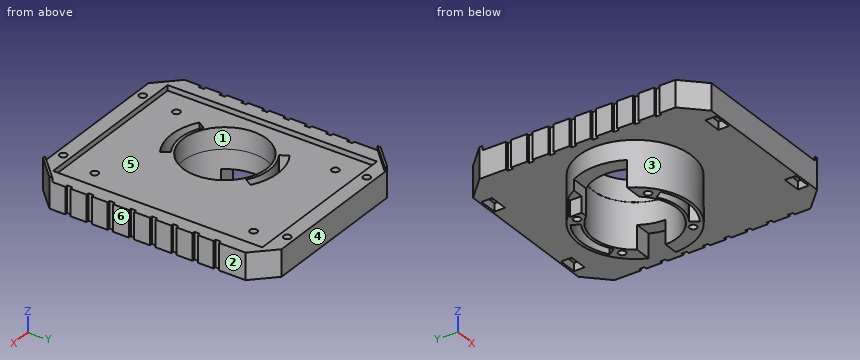
```python
from build123d import *

# Parameters (mm, degrees)
SKETCH1_W           = 92.71
SKETCH1_H           = 114.3
BOSS_EXTRUDE1_DEPTH = 12.7
SKETCH2_W           = 78.71000006
SKETCH2_H           = 100.30000006
CUT_EXTRUDE1_DEPTH  = 2.54
SKETCH3_R           = 19.939
CUT_EXTRUDE2_DEPTH  = 75.284144506
SKETCH4_R           = 26.9875
SKETCH4_R_2         = 19.98750003
BOSS_EXTRUDE2_DEPTH = 21.844
SKETCH6_R           = 1.750000056
CUT_EXTRUDE3_DEPTH  = 19.05
SKETCH12_W          = 12.7
SKETCH12_H          = 25.4
CUT_EXTRUDE6_DEPTH  = 77.759812799
SKETCH13_W          = 11.43
SKETCH13_H          = 11.43
CUT_EXTRUDE7_DEPTH  = 77.759812799
SKETCH14_R          = 1.750000056
CUT_EXTRUDE8_DEPTH  = 82.290814124
SKETCH16_W          = 8.89
SKETCH16_H          = 5.08
CUT_EXTRUDE9_DEPTH  = 3.81
SKETCH18_R          = 1.75
CUT_EXTRUDE11_DEPTH = 5.08
SKETCH19_W          = 2.54
SKETCH19_H          = 2.54
CUT_EXTRUDE12_DEPTH = 82.290814124
CHAMFER2_SIZE       = 10.16
CUT_EXTRUDE13_DEPTH = 82.290814124
BOSS_EXTRUDE3_DEPTH = 2
CUT_EXTRUDE14_START = -7.62
CUT_EXTRUDE14_DEPTH = 7.62


with BuildPart() as part:
    # Sketch1 → Boss-Extrude1 (new body)
    with BuildSketch(Plane.XY):
        Rectangle(SKETCH1_W, SKETCH1_H)
    extrude(amount=BOSS_EXTRUDE1_DEPTH)

    # Sketch2 → Cut-Extrude1 (cut)
    with BuildSketch(Plane.XY.offset(12.7)):
        Rectangle(SKETCH2_W, SKETCH2_H)
    extrude(amount=-CUT_EXTRUDE1_DEPTH, mode=Mode.SUBTRACT)

    # Sketch3 → Cut-Extrude2 (cut, through all)
    with BuildSketch(Plane.XY.offset(10.16)):
        with Locations((-13.335, -4.572)):
            Circle(SKETCH3_R)
    extrude(amount=-CUT_EXTRUDE2_DEPTH, mode=Mode.SUBTRACT)

    # Sketch4 → Boss-Extrude2 (add)
    with BuildSketch(Plane(origin=(0, 0, 0), x_dir=(-1, 0, 0), z_dir=(0, 0, -1))):
        with Locations((13.335, -4.572)):
            Circle(SKETCH4_R)
        with Locations((13.335, -4.572)):
            Circle(SKETCH4_R_2, mode=Mode.SUBTRACT)
    extrude(amount=BOSS_EXTRUDE2_DEPTH)

    # Sketch6 → Cut-Extrude3 (cut)
    with BuildSketch(Plane(origin=(0, 0, -21.844), x_dir=(-1, 0, 0), z_dir=(0, 0, -1))):
        with Locations((-2.11782644, 12.446)):
            Circle(SKETCH6_R)
        with Locations((28.78782644, -21.59)):
            Circle(SKETCH6_R)
        with Locations((28.78782644, 12.446)):
            Circle(SKETCH6_R)
        with Locations((-2.11782644, -21.59)):
            Circle(SKETCH6_R)
    extrude(amount=-CUT_EXTRUDE3_DEPTH, mode=Mode.SUBTRACT)

    # Sketch12 → Cut-Extrude6 (cut, through all)
    with BuildSketch(Plane(origin=(0, 0, 0), x_dir=(0, 0, -1), z_dir=(1, 0, 0))):
        with Locations((15.494, -4.572)):
            Rectangle(SKETCH12_W, SKETCH12_H)
    extrude(amount=-CUT_EXTRUDE6_DEPTH, mode=Mode.SUBTRACT)

    # Sketch13 → Cut-Extrude7 (cut, through all)
    with BuildSketch(Plane(origin=(0, 0, 0), x_dir=(0, 0, -1), z_dir=(1, 0, 0))):
        with Locations((16.129, 0.508)):
            Rectangle(SKETCH13_W, SKETCH13_H)
    extrude(amount=CUT_EXTRUDE7_DEPTH, mode=Mode.SUBTRACT)

    # Sketch14 → Cut-Extrude8 (cut, through all)
    with BuildSketch(Plane.XY.offset(12.7)):
        with Locations((-27.305, 53.65)):
            Circle(SKETCH14_R)
        with Locations((27.305, 53.65)):
            Circle(SKETCH14_R)
        with Locations((-27.305, -53.65)):
            Circle(SKETCH14_R)
        with Locations((27.305, -53.65)):
            Circle(SKETCH14_R)
    extrude(amount=-CUT_EXTRUDE8_DEPTH, mode=Mode.SUBTRACT)

    # Sketch16 → Cut-Extrude9 (cut)
    with BuildSketch(Plane(origin=(0, 0, 0), x_dir=(-1, 0, 0), z_dir=(0, 0, -1))):
        with Locations((-27.305, 53.65)):
            Rectangle(SKETCH16_W, SKETCH16_H)
        with Locations((27.305, 53.65)):
            Rectangle(SKETCH16_W, SKETCH16_H)
        with Locations((27.305, -53.65)):
            Rectangle(SKETCH16_W, SKETCH16_H)
        with Locations((-27.305, -53.65)):
            Rectangle(SKETCH16_W, SKETCH16_H)
    extrude(amount=-CUT_EXTRUDE9_DEPTH, mode=Mode.SUBTRACT)

    # Sketch18 → Cut-Extrude11 (cut)
    with BuildSketch(Plane.XY.offset(10.16)):
        with Locations((-28.17900003, 38.02150003)):
            Circle(SKETCH18_R)
        with Locations((27.92500003, 38.02150003)):
            Circle(SKETCH18_R)
        with Locations((-28.17900003, -38.14850003)):
            Circle(SKETCH18_R)
        with Locations((27.92500003, -38.14850003)):
            Circle(SKETCH18_R)
    extrude(amount=-CUT_EXTRUDE11_DEPTH, mode=Mode.SUBTRACT)

    # Sketch19 → Cut-Extrude12 (cut, through all)
    with BuildSketch(Plane.XY.offset(12.7)):
        with Locations((-46.355, -38.1)):
            Rectangle(SKETCH19_W, SKETCH19_H)
        with Locations((46.355, -38.1)):
            Rectangle(SKETCH19_W, SKETCH19_H)
        with Locations((-46.355, -27.94)):
            Rectangle(SKETCH19_W, SKETCH19_H)
        with Locations((46.355, -27.94)):
            Rectangle(SKETCH19_W, SKETCH19_H)
        with Locations((-46.355, -17.78)):
            Rectangle(SKETCH19_W, SKETCH19_H)
        with Locations((46.355, -17.78)):
            Rectangle(SKETCH19_W, SKETCH19_H)
        with Locations((-46.355, -7.62)):
            Rectangle(SKETCH19_W, SKETCH19_H)
        with Locations((46.355, -7.62)):
            Rectangle(SKETCH19_W, SKETCH19_H)
        with Locations((-46.355, 2.54)):
            Rectangle(SKETCH19_W, SKETCH19_H)
        with Locations((46.355, 2.54)):
            Rectangle(SKETCH19_W, SKETCH19_H)
        with Locations((-46.355, 12.7)):
            Rectangle(SKETCH19_W, SKETCH19_H)
        with Locations((46.355, 12.7)):
            Rectangle(SKETCH19_W, SKETCH19_H)
        with Locations((-46.355, 22.86)):
            Rectangle(SKETCH19_W, SKETCH19_H)
        with Locations((46.355, 22.86)):
            Rectangle(SKETCH19_W, SKETCH19_H)
        with Locations((-46.355, 33.02)):
            Rectangle(SKETCH19_W, SKETCH19_H)
        with Locations((46.355, 33.02)):
            Rectangle(SKETCH19_W, SKETCH19_H)
    extrude(amount=-CUT_EXTRUDE12_DEPTH, mode=Mode.SUBTRACT)

    # Chamfer2
    chamfer2_edges = [part.edges().sort_by_distance(p)[0] for p in [
        (46.355, -57.15, 6.35),
        (-46.355, -57.15, 6.35),
        (-46.355, 57.15, 6.35),
        (46.355, 57.15, 6.35),
    ]]
    chamfer(chamfer2_edges, length=CHAMFER2_SIZE)

    # Sketch20 → Cut-Extrude13 (cut, through all)
    with BuildSketch(Plane(origin=(0, 0, -21.844), x_dir=(-1, 0, 0), z_dir=(0, 0, -1))):
        with BuildLine():
            Line((-0.161794567, 17.099636308), (2.084843313, 13.492237618))
            ThreePointArc((2.084843313, 13.492237618), (13.335, 16.709041004), (24.585156687, 13.492237618))
            Line((24.585156687, 13.492237618), (26.831794567, 17.099636308))
            ThreePointArc((26.831794567, 17.099636308), (13.335, 20.958830066), (-0.161794567, 17.099636308))
        make_face()
        with BuildLine():
            Line((2.084843313, -22.636237618), (-0.161794567, -26.243636308))
            ThreePointArc((-0.161794567, -26.243636308), (13.335, -30.102830066), (26.831794567, -26.243636308))
            Line((26.831794567, -26.243636308), (24.585156687, -22.636237618))
            ThreePointArc((24.585156687, -22.636237618), (13.335, -25.853041004), (2.084843313, -22.636237618))
        make_face()
    extrude(amount=-CUT_EXTRUDE13_DEPTH, mode=Mode.SUBTRACT)

    # Sketch21 → Boss-Extrude3 (add)
    with BuildSketch(Plane.XY.offset(12.7)):
        Polygon((-40.567893219, 51.362893219), (-46.355, 45.575786438), (-46.355, 46.99), (-36.195, 57.15), (-34.780786438, 57.15), align=None)
        Polygon((40.567893219, -51.362893219), (34.780786438, -57.15), (36.195, -57.15), (46.355, -46.99), (46.355, -45.575786438), align=None)
    extrude(amount=BOSS_EXTRUDE3_DEPTH)

    # Sketch22 → Cut-Extrude14 (cut)
    with BuildSketch(Plane(origin=(0, 0, -21.844), x_dir=(-1, 0, 0), z_dir=(0, 0, -1)).offset(CUT_EXTRUDE14_START)):
        with BuildLine():
            Line((31.787826536, 8.128), (31.787826536, 13.716))
            Line((31.787826536, 13.716), (33.181264441, 13.716))
            ThreePointArc((33.181264441, 13.716), (35.342461556, 11.04839667), (37.1475, 8.128))
            Line((37.1475, 8.128), (31.787826536, 8.128))
        make_face()
    extrude(amount=CUT_EXTRUDE14_DEPTH, mode=Mode.SUBTRACT)


solid = part.part
```
For this review, take the finished solid that the model builds, in its own axes (mm). Face numbers are marked on the shaded views. A direction names the side the tool comes from. Round coordinates to 2 decimals unless told otherwise and drop trailing zeros. Write each loop counter-clockwise with the first axis right and the second up, starting at its lowest first coordinate (ties: lowest second). Pieces come first, ordered by that corner, then holes. Notation, with made-up numbers: (13.5, 10.5) -> (68.5, 10.5) arc R15 cw to (68.5, 39.5) -> close; hole circle Ø7 at (-11.75, -29). An arc over 180 degrees is marked (long way). Use one line per item in the form item = value.
1) Take a section at A-A, the plane z = -12.5. Count the separate pieces of the cut face and the enclosed holes in it, and give its area (3 significant figures).
Found:
separate_pieces = 2
enclosed_holes = 6
area = 502 mm2
2) Clearance check with flat-ended pins moving along their axes: pin 1 (2 mm diameter, centred on x = 37, y = 39, fed in from -Z); pin 2 (1 mm diameter, centred on x = -27.5, y = -38.5, fed in from +Z); pin 3 (5.5 mm diameter, centred on x = 10.5, z = -18.5, fed in from +Y). State where each tip first meets the part, or that it passes through.
Found:
pin_1 = 0
pin_2 = 5.08
pin_3 = 12.27
3) To check wall thickness, follow L1, parallel to Y at x = -29, z = -7.5; L2, parallel to X at y = -21, z = -14; L3, parallel to Y at x = -17, z = -9. State the ranges of each line that lie inside material, in increasing order. Write a range as from..to.
Found:
L1 = -26.55..-23.33, -19.85..-16.99, 7.84..10.71, 14.18..17.4
L2 = -34.75..-30.44, -27.14..-24.72, -1.95..0.47, 3.77..8.08
L3 = -31.31..-29.84, -25.54..-24.22, 15.08..16.39, 20.69..22.17
4) Take a section at B-B, the plane y = 53.65. Write out the cut boundary in (x, z) (3 decimals).
Found:
outline = (-39.695, 0) -> (-31.75, 0) -> (-31.75, 3.81) -> (-29.055, 3.81) -> (-29.055, 12.7) -> (-38.281, 12.7) -> (-38.281, 14.7) -> (-39.695, 14.7) -> close; (-25.555, 3.81) -> (-22.86, 3.81) -> (-22.86, 0) -> (22.86, 0) -> (22.86, 3.81) -> (25.555, 3.81) -> (25.555, 12.7) -> (-25.555, 12.7) -> close; (29.055, 3.81) -> (31.75, 3.81) -> (31.75, 0) -> (39.695, 0) -> (39.695, 12.7) -> (29.055, 12.7) -> close
5) Take a section at D-D, the plane y = 41. Write out the cut boundary in (x, z) (3 decimals), and give its area (3 significant figures).
Found:
outline = (-46.355, 0) -> (46.355, 0) -> (46.355, 12.7) -> (39.355, 12.7) -> (39.355, 10.16) -> (-39.355, 10.16) -> (-39.355, 12.7) -> (-46.355, 12.7) -> close
area = 977 mm2
6) Mouldability with a two-part tool opening along Y and no side actions: class the marked faces 1, 2, 3 and 4 as +Y half, -Y half, draft (parallel to the pull), parting line (faces both ways), or undercut.
Found:
face_1 = undercut
face_2 = draft
face_3 = parting line
face_4 = +Y half
7) Tool access review of the marked faces 5 and 6: name each direction out of +Z, -Z, +X, -X, +Y, -Y from which nothing blocks a thin tool from reaching the whole face with its end or side.
Found:
face_5 = +Z
face_6 = +Z, -Z, +X, +Y, -Y
